from build123d import *

# Parameters (mm, degrees)
SKETCH1_W           = 25.4
SKETCH1_H           = 32.3
BOSS_EXTRUDE1_DEPTH = 6.88
SKETCH3_R           = 111
SKETCH3_R_2         = 1.775
CUT_EXTRUDE1_DEPTH  = 6.88
CHAMFER1_SIZE       = 1.805302587
CHAMFER1_SIZE_2     = 2
FILLET1_R           = 2


with BuildPart() as part:
    # Sketch1 → Boss-Extrude1 (new body)
    with BuildSketch(Plane.XY):
        Rectangle(SKETCH1_W, SKETCH1_H)
    extrude(amount=BOSS_EXTRUDE1_DEPTH)

    # Sketch3 → Cut-Extrude1 (cut)
    with BuildSketch(Plane(origin=(0, 0, 0), x_dir=(-1, 0, 0), z_dir=(0, 0, -1))):
        with Locations((0, 113.850000001)):
            Circle(SKETCH3_R)
        with Locations((0, -3.149999999)):
            Circle(SKETCH3_R_2)
    extrude(amount=-CUT_EXTRUDE1_DEPTH, mode=Mode.SUBTRACT)

    # Chamfer1
    # the kernel refuses this chamfer: 2, 1.805302587 mm, written as the material it takes off along each edge
    with BuildSketch(Plane(origin=(-12.7, 3.578924918, 12.070681021), x_dir=(0, -1, 0), z_dir=(0, 0, -1))) as chamfer1_piece_1:
        with BuildLine():
            Line((CHAMFER1_SIZE, 0), (0.212697329, -2.007197118))
            ThreePointArc((0.212697329, -2.007197118), (0.113915873, -1.031505174), (0, 0))
            Line((0, 0), (CHAMFER1_SIZE, 0))
        make_face()
    extrude(amount=17.261362042, mode=Mode.SUBTRACT)
    with BuildSketch(Plane(origin=(12.7, 3.578924918, 12.070681021), x_dir=(0, -1, 0), z_dir=(0, 0, -1))) as chamfer1_piece_2:
        with BuildLine():
            Line((CHAMFER1_SIZE, 0), (0.212697329, 2.007197118))
            ThreePointArc((0.212697329, 2.007197118), (0.113915873, 1.031505174), (0, 0))
            Line((0, 0), (CHAMFER1_SIZE, 0))
        make_face()
    extrude(amount=17.261362042, mode=Mode.SUBTRACT)
    with BuildSketch(Plane(origin=(12.7, -16.15, -5.143365976), x_dir=(-1, 0, 0), z_dir=(0, 0, 1))) as chamfer1_piece_3:
        Polygon((CHAMFER1_SIZE_2, 0), (0, -CHAMFER1_SIZE_2), (0, 0), align=None)
    extrude(amount=17.166731952, mode=Mode.SUBTRACT)
    with BuildSketch(Plane(origin=(-12.7, -16.15, -5.143365976), x_dir=(1, 0, 0), z_dir=(0, 0, 1))) as chamfer1_piece_4:
        Polygon((CHAMFER1_SIZE_2, 0), (0, CHAMFER1_SIZE_2), (0, 0), align=None)
    extrude(amount=17.166731952, mode=Mode.SUBTRACT)

    # Fillet1
    fillet1_edges = [part.edges().sort_by_distance(p)[0] for p in [
        (12.7, -14.15, 3.44),
        (12.7, 1.773622331, 3.44),
        (-10.692802882, 3.366227588, 3.44),
        (10.692802882, 3.366227588, 3.44),
        (-10.7, -16.15, 3.44),
        (10.7, -16.15, 3.44),
        (-12.7, -14.15, 3.44),
        (-12.7, 1.773622331, 3.44),
    ]]
    fillet(fillet1_edges, radius=FILLET1_R)


solid = part.part
Geometry: final body of the model. Coordinates: model frame, mm. Round coordinates to 2 decimals unless told otherwise and drop trailing zeros. Loops run counter-clockwise (first coordinate to the right, second up) from the corner with the lowest first, then second, coordinate; pieces in that order, holes last.
Q1. Material intervals for L1, parallel to Y at x = -1, z = 3.5; L2, parallel to X at y = -14.75, z = 2; L3, parallel to Y at x = 8, z = 0.5, sorted ascending.
Q2. Section D-D on x = -3.5. Return loops of the section in (y, z), plus the area to 3 significant figures.
Q3. Section B-B on x = 0. Return loops of the section in (y, z) (3 decimals), plus the area to 3 significant figures.
Q4. Section A-A on y = -3.15. Return loops of the section in (x, z) (3 decimals), plus the area to 3 significant figures.
Q5. Section C-C on z = 2.5. Return loops of the section in (x, y) (3 decimals), plus the area to 3 significant figures.
Q6. Pull-direction query (X, two-part tool) for faces 1 (the cylindrical face through (0.14, 2.85, 3.39)), 2 (the flat face through (11.69, -15.16, 3.39)), 3 (the cylindrical face through (0.23, -1.39, 3.39)), 4 (the flat face through (-12.7, -6, 3)); classes: released by +X, released by -X, zero draft, split by the parting line, or undercut.
Evaluation:
1. L1: y = -16.15 to -4.62, -1.68 to 2.85
1. L2: x = -12.1 to 12.1
1. L3: y = -16.15 to 3.14
2. outline: (-16.15, 0) - (2.91, 0) - (2.91, 6.88) - (-16.15, 6.88) - close
2. area: 131 mm2
3. outline: (-16.15, 0) - (-4.925, 0) - (-4.925, 6.88) - (-16.15, 6.88) - close; (-1.375, 0) - (2.85, 0) - (2.85, 6.88) - (-1.375, 6.88) - close
3. area: 106 mm2
4. outline: (-12.7, 0) - (-1.775, 0) - (-1.775, 6.88) - (-12.7, 6.88) - close; (1.775, 0) - (12.7, 0) - (12.7, 6.88) - (1.775, 6.88) - close
4. area: 150 mm2
5. outline: (-12.7, -13.322) arc R2 ccw to (-12.114, -14.736) - (-11.286, -15.564) arc R2 ccw to (-9.872, -16.15) - (9.872, -16.15) arc R2 ccw to (11.286, -15.564) - (12.114, -14.736) arc R2 ccw to (12.7, -13.322) - (12.7, 0.807) arc R2 ccw to (11.943, 2.374) - (11.322, 2.867) arc R2 ccw to (9.9, 3.292) arc R111 cw to (-9.9, 3.292) arc R2 ccw to (-11.322, 2.867) - (-11.943, 2.374) arc R2 ccw to (-12.7, 0.807) - close; hole circle Ø3.55 at (0, -3.15)
5. area: 470 mm2
6. face 1: undercut
6. face 2: released by +X
6. face 3: undercut
6. face 4: released by -X
